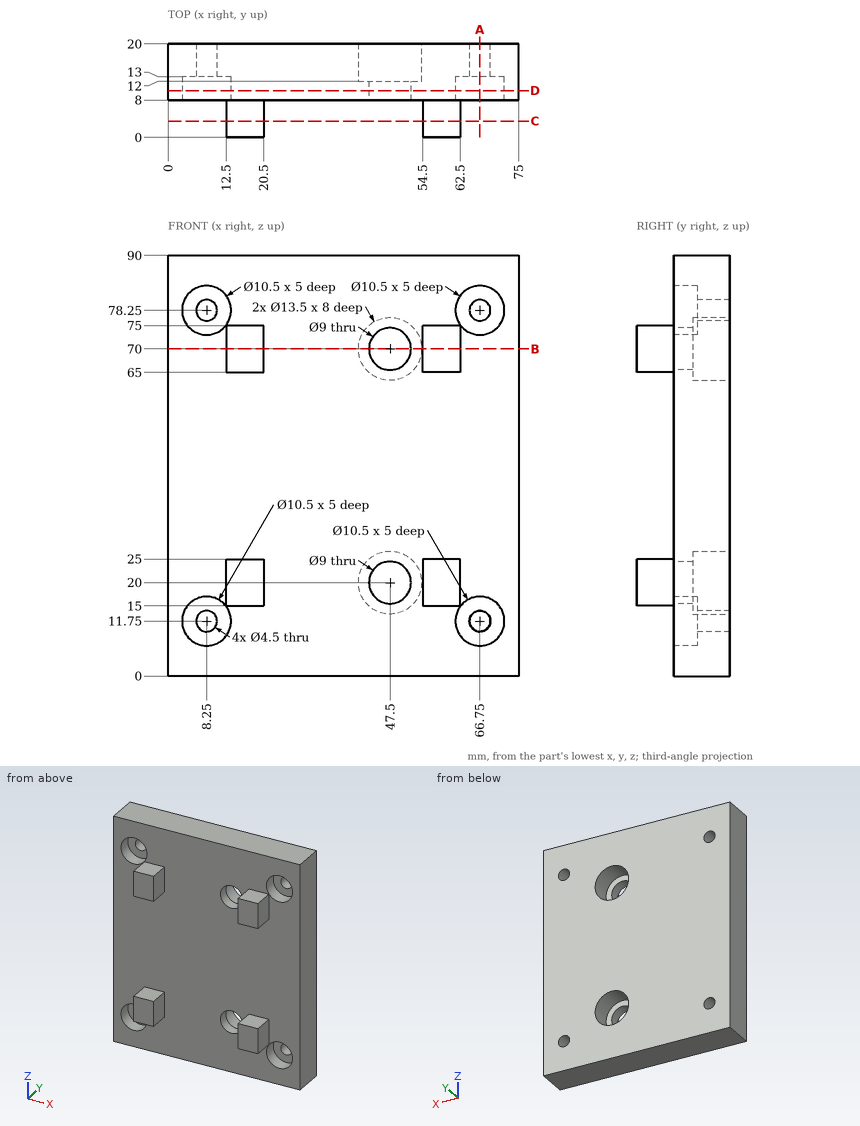
Part print with two shaded views. Sizes in mm from the minimum x, y, z corner. Give positions to 0.01 mm unless a question says otherwise; leave off trailing zeros. Order: outer loops, then holes, each group sorted by start corner. A loop starts at its lowest first (then second) coordinate and runs counter-clockwise, first axis right, second up. Notation, with made-up numbers: M 73,78 L 95,78 A10 ccw 95,88 Z; hole C 18,5.5 d8. An arc over 180 degrees is marked long. Use one line per item in the form item = value.
1) Saw through at D-D (y = 10). Give the cut face in (x, z), plus the area to 3 significant figures.
Calculated:
outline = M 0,0 L 75,0 L 75,90 L 0,90 Z; hole C 8.25,11.75 d10.5; hole C 8.25,78.25 d10.5; hole C 47.5,20 d9; hole C 47.5,70 d9; hole C 66.75,11.75 d10.5; hole C 66.75,78.25 d10.5
area = 6,280 mm2
2) Saw through at A-A (x = 66.75). Give the cut face in (y, z), plus the area to 3 significant figures.
Calculated:
outline = M 8,0 L 20,0 L 20,9.5 L 13,9.5 L 13,6.5 L 8,6.5 Z; M 8,17 L 13,17 L 13,14 L 20,14 L 20,76 L 13,76 L 13,73 L 8,73 Z; M 8,83.5 L 13,83.5 L 13,80.5 L 20,80.5 L 20,90 L 8,90 Z
area = 912 mm2
3) Saw through at C-C (y = 3.5). Give the cut face in (x, z), plus the area to 3 significant figures.
Calculated:
outline = M 12.5,15 L 20.5,15 L 20.5,25 L 12.5,25 Z; M 12.5,65 L 20.5,65 L 20.5,75 L 12.5,75 Z; M 54.5,15 L 62.5,15 L 62.5,25 L 54.5,25 Z; M 54.5,65 L 62.5,65 L 62.5,75 L 54.5,75 Z
area = 320 mm2
4) Saw through at B-B (z = 70). Give the cut face in (x, y).
Calculated:
outline = M 0,8 L 12.5,8 L 12.5,0 L 20.5,0 L 20.5,8 L 43,8 L 43,12 L 40.75,12 L 40.75,20 L 0,20 Z; M 52,8 L 54.5,8 L 54.5,0 L 62.5,0 L 62.5,8 L 75,8 L 75,20 L 54.25,20 L 54.25,12 L 52,12 Z
5) Drop flat-ended pins along their axis: pin 1 (6.5 mm diameter, centred on y = 2.5, z = 21.5, fed in from +X); pin 2 (1 mm diameter, centred on y = 5, z = 19, fed in from -X); pin 3 (4 mm diameter, centred on y = 17, z = 66.5, fed in from -X); pin 4 (9 mm diameter, centred on x = 58.5, y = 2.5, fed in from -Z). Give the stop position or say it passes through.
Calculated:
pin_1 = 62.5
pin_2 = 12.5
pin_3 = 0
pin_4 = 15
6) Probe probe 1 along Z at (x, y) = (47.5, 10.4); probe 2 along Z at (x, y) = (66.75, 10.15); probe 3 along Y at (x, z) = (14, 27). List the from-to ranges inside material, lowest first.
Calculated:
probe_1 = 0 to 15.5, 24.5 to 65.5, 74.5 to 90
probe_2 = 0 to 6.5, 17 to 73, 83.5 to 90
probe_3 = 8 to 20
